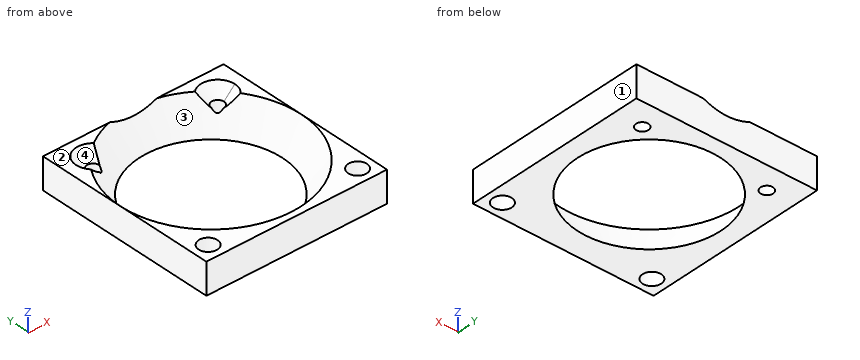
from build123d import *

# Parameters (mm, degrees)
F0_W        = 29
F0_H        = 29.5
F0_R        = 1.5
F0_R_2      = 1
F0_R_3      = 11.5
F1_DEPTH    = 5
F4_T2_ANGLE = 359.64
F4_T4_ANGLE = 359.64
F4_T6_ANGLE = 359.64


# Not quite as in the source:
# - a fillet or chamfer that OpenCascade refuses, or shapes differently, is made with other operations: its cross-section is extruded or revolved along the edge and cut away or added


with BuildPart() as f1:
    # F0 (on Top) → F1 (new body)
    with BuildSketch(Plane.XY):
        with Locations((0, -0.75)):
            Rectangle(F0_W, F0_H)
        with Locations((-12, -13)):
            Circle(F0_R, mode=Mode.SUBTRACT)
        with Locations((12, -13)):
            Circle(F0_R, mode=Mode.SUBTRACT)
        with Locations((-10, 10)):
            Circle(F0_R_2, mode=Mode.SUBTRACT)
        Circle(F0_R_3, mode=Mode.SUBTRACT)
        with Locations((10, 10)):
            Circle(F0_R_2, mode=Mode.SUBTRACT)
    extrude(amount=F1_DEPTH)

    # F2 (on Right) → F3 (revolve, cut)
    with BuildSketch(Plane.YZ):
        Polygon((-14.5, 5), (-11.5, 0), (-11.5, 5), align=None)
    revolve(axis=Axis((0, 0, 6.3592060469), (0, 0, 1)), mode=Mode.SUBTRACT)

    # F4: chamfer of 1.75 on 3 edges, made by hand

    # F4_s1 → F4_t2 (revolve, cut)
    with BuildSketch(Plane(origin=(0.0313170241, 0.0315144155, 0), x_dir=(0, 0, 1), z_dir=(-0.7048818539, -0.7093247296, 0))):
        Polygon((3.25, 13.1420658351), (5, 11.3920658351), (5, 13.1420658351), align=None)
    revolve(axis=Axis((-10, 10, 5), (0, 0, 1)), revolution_arc=F4_T2_ANGLE, mode=Mode.SUBTRACT)

    # F4_s3 → F4_t4 (revolve, cut)
    with BuildSketch(Plane(origin=(-0.0624354204, 9.9367750216, 0), x_dir=(0, 0, 1), z_dir=(0.006283144, -0.9999802609, 0))):
        Polygon((5, -12.8126340482), (3.25, -11.0626340482), (5, -11.0626340482), align=None)
    revolve(axis=Axis((10, 10, 5), (0, 0, 1)), revolution_arc=F4_T4_ANGLE, mode=Mode.SUBTRACT)

    # F4_s5 → F4_t6 (revolve, cut)
    with BuildSketch(Plane.XZ.offset(-10)):
        Polygon((12.75, 5), (11, 3.25), (11, 5), align=None)
    revolve(axis=Axis((10, 10, 5), (0, 0, 1)), revolution_arc=F4_T6_ANGLE, mode=Mode.SUBTRACT)


solid = f1.part
For this review, take the finished solid that the model builds, in its own axes (mm). Face numbers are marked on the shaded views. Round coordinates to 2 decimals unless told otherwise and drop trailing zeros. Write each loop counter-clockwise with the first axis right and the second up, starting at its lowest first coordinate (ties: lowest second). Pieces come first, ordered by that corner, then holes. Notation, with made-up numbers: (-19.75, 88) - (2.25, 88) arc R16 ccw to (2.25, 97) - close; hole circle Ø2 at (-5, -38). An arc over 180 degrees is marked (long way). Write item = value, one per line. Start each with the question number.
1. For pin 1 Ø3 at (x, y) = (10, 10) entering from +Z, flat-tipped, find the tip position at first contact; note if it passes through.
2. Wall thickness on L1, parallel to Y at x = -11.75, z = 2.15; L2, parallel to X at y = 10, z = 1.85; L3, parallel to Y at x = -12, z = 4.15: over which ranges is each line inside the solid? List them lowest first.
3. Consider section B-B on x = 0. State the section outline as (y, z) points.
4. Consider section A-A on z = 1.55. State the section outline as (x, y) points.
5. Draft analysis for pull direction X (two halves, no side actions). For the marked faces 1, 2, 3 and 4, state which applies: released by +X, released by -X, zero draft, split by the parting line, or undercut.
Evaluation:
q1.pin_1 = 3.75
q2.L1 = -15.5 to -14.48, -11.52 to -5.05, 5.05 to 14
q2.L2 = -14.5 to -11, -9 to -7.68, 7.68 to 9, 11 to 14.5
q2.L3 = -15.5 to -14.5, -11.5 to -7.19, 7.19 to 14
q3.outline = (-15.5, 0) - (-11.5, 0) - (-14.5, 5) - (-15.5, 5) - close; (11.5, 0) - (14, 0) - (14, 4.17) - close
q4.outline = (-14.5, -15.5) - (14.5, -15.5) - (14.5, 14) - (-14.5, 14) - close; hole circle Ø3 at (-12, -13); hole circle Ø24.86 at (0, 0); hole circle Ø2 at (-10, 10); hole circle Ø2 at (10, 10); hole circle Ø3 at (12, -13)
q5.face_1 = released by +X
q5.face_2 = zero draft
q5.face_3 = undercut
q5.face_4 = undercut
